from build123d import *

# Parameters (mm, degrees)
SKETCH_1_R          = 5.98
EXTRUDE_1_DEPTH     = 0.2
SKETCH_2_R          = 2.8
EXTRUDE_2_DEPTH     = 0.9
SKETCH_3_R          = 5.98
EXTRUDE_3_DEPTH     = 1
EXTRUDE_START       = -0.6
SKETCH_4_R          = 5.98
EXTRUDE_4_DEPTH     = 0.6
CUT_EXTRUDE_START   = -0.2
SKETCH_6_R          = 3.55
SKETCH_6_R_2        = 2.8
CUT_EXTRUDE_2_DEPTH = 0.2
EXTRUDE_START_2     = 6
SKETCH_7_R          = 5.98
SKETCH_7_R_2        = 5.25
EXTRUDE_5_DEPTH     = 6
CHAMFER_4_SIZE      = 1
CHAMFER_5_SIZE      = 0.4
CHAMFER_6_SIZE      = 0.4
CHAMFER_7_SIZE      = 1


with BuildPart() as part:
    # Sketch 1 → Extrude 1 (new body)
    with BuildSketch(Plane.XY):
        Circle(SKETCH_1_R)
        with BuildLine():
            Line((-0.6, 5.25), (0, 5.85))
            Line((0, 5.85), (0.6, 5.25))
            Line((0.6, 5.25), (0.6, 1.670516387))
            ThreePointArc((0.6, 1.670516387), (0.8875, 1.537195092), (1.146709629, 1.354873436))
            Line((1.146709629, 1.354873436), (4.24663337, 3.144615242))
            Line((4.24663337, 3.144615242), (5.066248612, 2.925))
            Line((5.066248612, 2.925), (4.84663337, 2.105384758))
            Line((4.84663337, 2.105384758), (1.746709629, 0.315642951))
            ThreePointArc((1.746709629, 0.315642951), (1.76791326, 0.158454108), (1.775, 0))
            ThreePointArc((1.775, 0), (1.76791326, -0.158454108), (1.746709629, -0.315642951))
            Line((1.746709629, -0.315642951), (4.84663337, -2.105384758))
            Line((4.84663337, -2.105384758), (5.066248612, -2.925))
            Line((5.066248612, -2.925), (4.24663337, -3.144615242))
            Line((4.24663337, -3.144615242), (1.146709629, -1.354873436))
            ThreePointArc((1.146709629, -1.354873436), (0.8875, -1.537195092), (0.6, -1.670516387))
            Line((0.6, -1.670516387), (0.6, -5.25))
            Line((0.6, -5.25), (0, -5.85))
            Line((0, -5.85), (-0.6, -5.25))
            Line((-0.6, -5.25), (-0.6, -1.670516387))
            ThreePointArc((-0.6, -1.670516387), (-0.8875, -1.537195092), (-1.146709629, -1.354873436))
            Line((-1.146709629, -1.354873436), (-4.24663337, -3.144615242))
            Line((-4.24663337, -3.144615242), (-5.066248612, -2.925))
            Line((-5.066248612, -2.925), (-4.84663337, -2.105384758))
            Line((-4.84663337, -2.105384758), (-1.746709629, -0.315642951))
            ThreePointArc((-1.746709629, -0.315642951), (-1.775, 0), (-1.746709629, 0.315642951))
            Line((-1.746709629, 0.315642951), (-4.84663337, 2.105384758))
            Line((-4.84663337, 2.105384758), (-5.066248612, 2.925))
            Line((-5.066248612, 2.925), (-4.24663337, 3.144615242))
            Line((-4.24663337, 3.144615242), (-1.146709629, 1.354873436))
            ThreePointArc((-1.146709629, 1.354873436), (-0.8875, 1.537195092), (-0.6, 1.670516387))
            Line((-0.6, 1.670516387), (-0.6, 5.25))
        make_face(mode=Mode.SUBTRACT)
    extrude(amount=EXTRUDE_1_DEPTH)

    # Sketch 3 → Extrude 3 (add)
    with BuildSketch(Plane.XY.offset(0.2)):
        Circle(SKETCH_3_R)
        with BuildLine():
            Line((-4.933776406, -2.430606997), (-5.066248612, -2.925))
            Line((-5.066248612, -2.925), (-4.571855609, -3.057472206))
            ThreePointArc((-4.571855609, -3.057472206), (-2.75, -4.763139721), (-0.361920797, -5.488079203))
            Line((-0.361920797, -5.488079203), (0, -5.85))
            Line((0, -5.85), (0.361920797, -5.488079203))
            ThreePointArc((0.361920797, -5.488079203), (2.75, -4.763139721), (4.571855609, -3.057472206))
            Line((4.571855609, -3.057472206), (5.066248612, -2.925))
            Line((5.066248612, -2.925), (4.933776406, -2.430606997))
            ThreePointArc((4.933776406, -2.430606997), (5.5, 0), (4.933776406, 2.430606997))
            Line((4.933776406, 2.430606997), (5.066248612, 2.925))
            Line((5.066248612, 2.925), (4.571855609, 3.057472206))
            ThreePointArc((4.571855609, 3.057472206), (2.75, 4.763139721), (0.361920797, 5.488079203))
            Line((0.361920797, 5.488079203), (0, 5.85))
            Line((0, 5.85), (-0.361920797, 5.488079203))
            ThreePointArc((-0.361920797, 5.488079203), (-2.75, 4.763139721), (-4.571855609, 3.057472206))
            Line((-4.571855609, 3.057472206), (-5.066248612, 2.925))
            Line((-5.066248612, 2.925), (-4.933776406, 2.430606997))
            ThreePointArc((-4.933776406, 2.430606997), (-5.5, 0), (-4.933776406, -2.430606997))
        make_face(mode=Mode.SUBTRACT)
    extrude(amount=EXTRUDE_3_DEPTH)



with BuildPart() as body_2:
    # Sketch 2 → Extrude 2 (new body)
    with BuildSketch(Plane.XY):
        Circle(SKETCH_2_R)
    extrude(amount=EXTRUDE_2_DEPTH)


with BuildPart() as part_1:
    add(part.part)

    add(body_2.part)  # Extrude 4 merges body 2
    # Sketch 4 → Extrude 4 (add)
    with BuildSketch(Plane.XY.offset(EXTRUDE_START)):
        Circle(SKETCH_4_R)
    extrude(amount=EXTRUDE_4_DEPTH)

    # Sketch 6 → Cut-Extrude 2 (cut)
    with BuildSketch(Plane.XY.offset(0.2).offset(CUT_EXTRUDE_START)):
        Circle(SKETCH_6_R)
        Circle(SKETCH_6_R_2, mode=Mode.SUBTRACT)
    extrude(amount=CUT_EXTRUDE_2_DEPTH, mode=Mode.SUBTRACT)

    # Sketch 7 → Extrude 5 (add)
    with BuildSketch(Plane(origin=(0, 0, -0.6), x_dir=(-1, 0, 0), z_dir=(0, 0, -1)).offset(EXTRUDE_START_2)):
        with Locations(Location((0, 0, 0), (0, 0, 180))):
            Circle(SKETCH_7_R)
        Circle(SKETCH_7_R_2, mode=Mode.SUBTRACT)
    extrude(amount=-EXTRUDE_5_DEPTH)

    # Chamfer 4
    chamfer_4_edges = [part_1.edges().sort_by_distance(p)[0] for p in [
        (5.25, 0, -0.6),
    ]]
    chamfer(chamfer_4_edges, length=CHAMFER_4_SIZE)

    # Chamfer 5
    # the kernel refuses this chamfer: 0.4 mm, written as the material it takes off along each edge
    with BuildSketch(Plane(origin=(0, 0, 1.2), x_dir=(1, 0, 0), z_dir=(0, -1, 0))) as chamfer_5_piece_1:
        Polygon((5.98, -CHAMFER_5_SIZE), (5.98 - CHAMFER_5_SIZE, 0), (5.98, 0), align=None)
    revolve(axis=Axis((0, 0, 1.2), (0, 0, 1)), mode=Mode.SUBTRACT)

    # Chamfer 6
    chamfer_6_edges = [part_1.edges().sort_by_distance(p)[0] for p in [
        (-5.98, 0, -6.6),
    ]]
    chamfer(chamfer_6_edges, length=CHAMFER_6_SIZE)

    # Chamfer 7
    # the kernel refuses this chamfer: 1 mm, written as the material it takes off along each edge
    with BuildSketch(Plane(origin=(0, 0, 0.9), x_dir=(1, 0, 0), z_dir=(0, -1, 0))) as chamfer_7_piece_1_section:
        Polygon((2.8, -CHAMFER_7_SIZE), (2.8 - CHAMFER_7_SIZE, 0), (2.8, 0), align=None)
    chamfer_7_piece_1 = revolve(axis=Axis((0, 0, 0.9), (0, 0, 1)), mode=Mode.PRIVATE)
    chamfer_7_piece_1 = split(chamfer_7_piece_1, bisect_by=Plane(origin=(-2.250209939, 0, 0), z_dir=(0, 0, 1)), keep=Keep.TOP, mode=Mode.PRIVATE)
    add(chamfer_7_piece_1, mode=Mode.SUBTRACT)


solid = part_1.part
Source: CAD feature listing. Evaluate the final solid. Frame: model axes, mm. A direction names the side the tool comes from. Coordinates: 2 decimals unless noted, no trailing zeros. Order: outer loops, then holes, each group sorted by start corner. A loop starts at its lowest first (then second) coordinate and runs counter-clockwise, first axis right, second up. Notation, with made-up numbers: M 53.5,-3 L 61.5,-3 A17 ccw 61.5,15 Z; hole C 27.25,18.5 d1. An arc over 180 degrees is marked long. Write each question's results on one line, items separated by ' | '. Start each with the question number.
1. Draft query along Y for faces 3 (the face through (5.5, 0, 0.7)), 4 (the face through (0, 0, 0.9)). Return one class per face: +Y half, -Y half, draft (parallel to the pull), parting line (faces both ways), or undercut.
2. Pin query (flat end, axial travel): pin 1 (1.7 mm diameter, centred on x = 4.5, y = -1, fed in from +Z); pin 2 (3 mm diameter, centred on x = -1, y = 0, fed in from +Z). Return the tip coordinate at first contact, or that it passes through.
3. Section C-C, the plane z = -5. Return the cut outline in (x, y).
4. Section B-B, the plane y = 0. Return the cut outline in (x, z), then the cut area to 3 significant figures.
5. Reachability of faces 1 (the face through (-4, 0, 0.2)), 2 (the face through (0, 0, -0.6)) from +Z, -Z, +X, -X, +Y, -Y: full face, straight path, thin tool, end or side. Return the list, or none.
6. Material intervals for L1, parallel to Y at x = 0, z = -4.5; L2, parallel to Y at x = -4.5, z = 0.5; L3, parallel to Z at x = -0.25, y = -3.25, sorted ascending.
7. Section A-A, the plane z = 0.5. Return the cut outline in (x, y) (3 decimals).
Solution:
1) face 3: undercut | face 4: undercut
2) pin 1: z = 0.2 | pin 2: z = 0.9
3) outline: C 0,0 d11.96; hole C 0,0 d10.5
4) outline: M -5.98,-6.2 L -5.58,-6.6 L -5.25,-6.6 L -5.25,-1.6 L -4.25,-0.6 L 4.25,-0.6 L 5.25,-1.6 L 5.25,-6.6 L 5.58,-6.6 L 5.98,-6.2 L 5.98,0.8 L 5.58,1.2 L 5.5,1.2 L 5.5,0.2 L 3.55,0.2 L 3.55,0 L 2.7,0 L 1.8,0.9 L -1.8,0.9 L -2.7,0 L -3.55,0 L -3.55,0.2 L -5.5,0.2 L -5.5,1.2 L -5.58,1.2 L -5.98,0.8 Z | area: 22.6 mm²
5) face 1: +Z | face 2: -Z
6) L1: -5.98 to -5.25, 5.25 to 5.98 | L2: -3.94 to -3.16, 3.16 to 3.94 | L3: -0.6 to 0
7) outline: C 0,0 d11.96; C 0,0 d4.4; hole M -5.066,-2.925 L -4.572,-3.057 A5.5 ccw -0.362,-5.488 L 0,-5.85 L 0.362,-5.488 A5.5 ccw 4.572,-3.057 L 5.066,-2.925 L 4.934,-2.431 A5.5 ccw 4.934,2.431 L 5.066,2.925 L 4.572,3.057 A5.5 ccw 0.362,5.488 L 0,5.85 L -0.362,5.488 A5.5 ccw -4.572,3.057 L -5.066,2.925 L -4.934,2.431 A5.5 ccw -4.934,-2.431 Z
